Can you work these out from the drawing? Everything is in mm from the part's minimum corner. Coordinates: 2 decimals unless noted, no trailing zeros. Order: outer loops, then holes, each group sorted by start corner. A loop starts at its lowest first (then second) coordinate and runs counter-clockwise, first axis right, second up. Notation, with made-up numbers: (-23, -10.5) - (16, -10.5) arc R35 ccw to (16, 22.5) - close; hole circle Ø4 at (62, 21). An arc over 180 degrees is marked (long way). One line per item, written item: value.
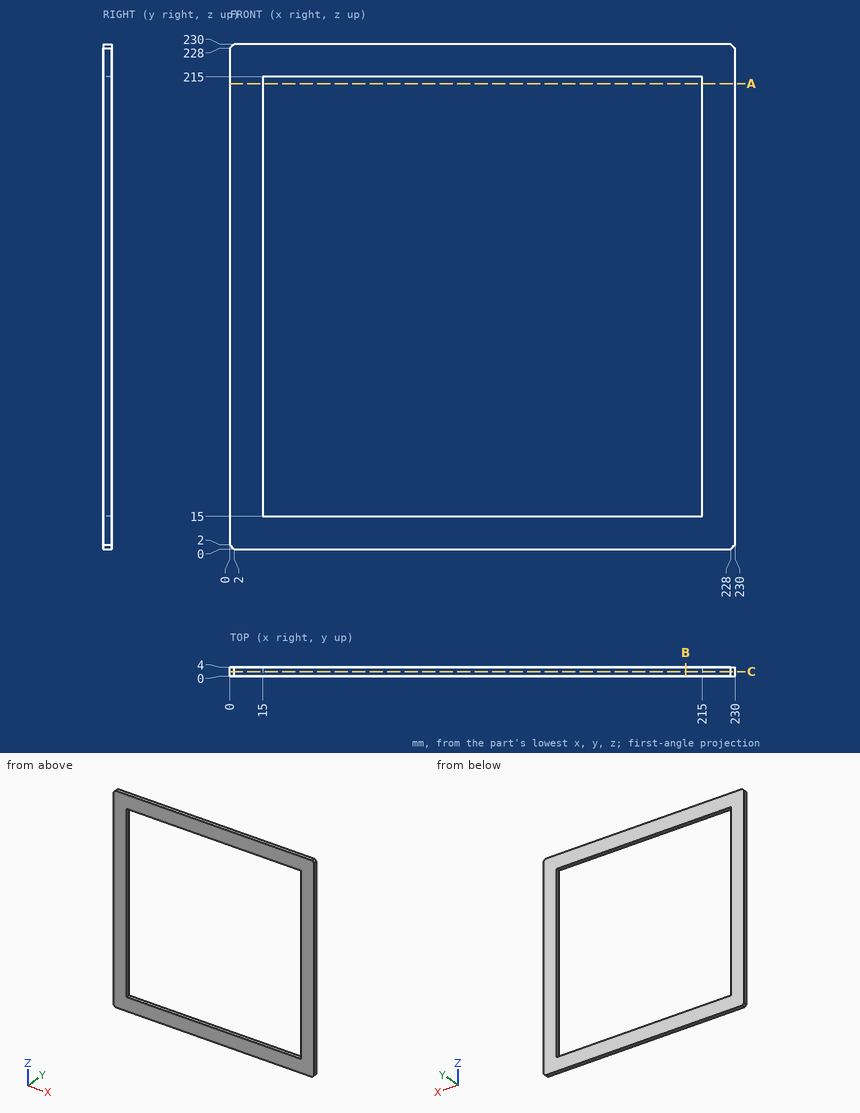
Item 1: I want a section at A-A on z = 212. Please give me the cut outline in (x, y), then the cut area to 3 significant figures.
Conclusion:
outline: (0, 0) - (15, 0) - (15, 4) - (0, 4) - close; (215, 0) - (230, 0) - (230, 4) - (215, 4) - close
area: 120 mm²
Item 2: If I drill on probe 1 along X at (y, z) = (1.75, 108.5), over which ranges is the centre line in solid material (lowest first)?
Conclusion:
probe 1: 0 to 15, 215 to 230
Item 3: I want a section at B-B on x = 207.5. Please give me the cut outline in (y, z), then the cut area to 3 significant figures.
Conclusion:
outline: (0, 0) - (4, 0) - (4, 15) - (0, 15) - close; (0, 215) - (4, 215) - (4, 230) - (0, 230) - close
area: 120 mm²
Item 4: I want a section at C-C on y = 2. Please give me the cut outline in (x, z), then the cut area to 3 significant figures.
Conclusion:
outline: (0, 2) - (2, 0) - (228, 0) - (230, 2) - (230, 228) - (228, 230) - (2, 230) - (0, 228) - close; hole (15, 15) - (215, 15) - (215, 215) - (15, 215) - close
area: 12,900 mm²
